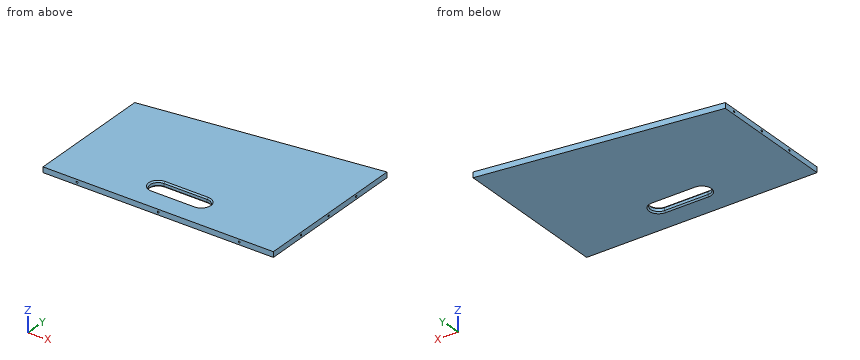
```python
from build123d import *

# Parameters (mm, degrees)
BOSS_EXTRUDE1_DEPTH       = 10
CUT_EXTRUDE1_DEPTH        = 516.437678095
CHAMFER1_SIZE             = 2.5
M4X0_7_TAPPED_HOLE1_D     = 3.3
M4X0_7_TAPPED_HOLE1_DEPTH = 12
M4X0_7_TAPPED_HOLE1_TIP   = 0.991420021
M4X0_7_TAPPED_HOLE2_D     = 3.3
M4X0_7_TAPPED_HOLE2_DEPTH = 12
M4X0_7_TAPPED_HOLE2_TIP   = 0.991420021
M4X0_7_TAPPED_HOLE3_D     = 3.3
M4X0_7_TAPPED_HOLE3_DEPTH = 12
M4X0_7_TAPPED_HOLE3_TIP   = 0.991420021


with BuildPart() as part:
    # Sketch1 → Boss-Extrude1 (new body)
    with BuildSketch(Plane.XY):
        Polygon((0, 234), (0, 290), (-426, 234), (-426, 0), (0, 0), align=None)
    extrude(amount=BOSS_EXTRUDE1_DEPTH)

    # Sketch2 → Cut-Extrude1 (cut, through all)
    with BuildSketch(Plane(origin=(0, 0, 0), x_dir=(-1, 0, 0), z_dir=(0, 0, -1))):
        with BuildLine():
            Line((173, 70), (253, 70))
            ThreePointArc((253, 70), (268, 55), (253, 40))
            Line((253, 40), (173, 40))
            ThreePointArc((173, 40), (158, 55), (173, 70))
        make_face()
    extrude(amount=-CUT_EXTRUDE1_DEPTH, mode=Mode.SUBTRACT)

    # Chamfer1
    chamfer1_edges = [part.edges().sort_by_distance(p)[0] for p in [
        (-268, 55, 10),
        (-213, 40, 10),
        (-158, 55, 10),
        (-213, 70, 10),
        (-268, 55, 0),
        (-213, 70, 0),
        (-158, 55, 0),
        (-213, 40, 0),
    ]]
    chamfer(chamfer1_edges, length=CHAMFER1_SIZE)

    # M4x0.7 Tapped Hole1
    with Locations(Plane(origin=(0, 0, 0), x_dir=(-1, 0, 0), z_dir=(0, -1, 0))):
        with Locations((63, -5), (213, -5), (363, -5)):
            Hole(M4X0_7_TAPPED_HOLE1_D / 2, depth=M4X0_7_TAPPED_HOLE1_DEPTH)
            with Locations((0, 0, -(M4X0_7_TAPPED_HOLE1_DEPTH + M4X0_7_TAPPED_HOLE1_TIP / 2))):  # 118° drill point
                Cone(0, M4X0_7_TAPPED_HOLE1_D / 2, M4X0_7_TAPPED_HOLE1_TIP, mode=Mode.SUBTRACT)

    # M4x0.7 Tapped Hole2
    with Locations(Plane.ZY.offset(426)):
        with Locations((5, 70.5), (5, 141), (5, 211.5)):
            Hole(M4X0_7_TAPPED_HOLE2_D / 2, depth=M4X0_7_TAPPED_HOLE2_DEPTH)
            with Locations((0, 0, -(M4X0_7_TAPPED_HOLE2_DEPTH + M4X0_7_TAPPED_HOLE2_TIP / 2))):  # 118° drill point
                Cone(0, M4X0_7_TAPPED_HOLE2_D / 2, M4X0_7_TAPPED_HOLE2_TIP, mode=Mode.SUBTRACT)

    # M4x0.7 Tapped Hole3
    with Locations(Plane(origin=(0, 0, 0), x_dir=(0, 0, -1), z_dir=(1, 0, 0))):
        with Locations((-5, 70.5), (-5, 141), (-5, 211.5)):
            Hole(M4X0_7_TAPPED_HOLE3_D / 2, depth=M4X0_7_TAPPED_HOLE3_DEPTH)
            with Locations((0, 0, -(M4X0_7_TAPPED_HOLE3_DEPTH + M4X0_7_TAPPED_HOLE3_TIP / 2))):  # 118° drill point
                Cone(0, M4X0_7_TAPPED_HOLE3_D / 2, M4X0_7_TAPPED_HOLE3_TIP, mode=Mode.SUBTRACT)


solid = part.part
```
Read the model definition and answer for the solid it produces. Units are mm, in the model's axes. Round coordinates to 2 decimals unless told otherwise and drop trailing zeros. Write each loop counter-clockwise with the first axis right and the second up, starting at its lowest first coordinate (ties: lowest second). Pieces come first, ordered by that corner, then holes. Notation, with made-up numbers: (19.5, -36) - (49.5, -36) arc R9 ccw to (49.5, -26) - close; hole circle Ø5 at (37.5, 28). An arc over 180 degrees is marked (long way). Use CSV: the item, a comma, the result in double quotes.
Q1. Find section A-A, the plane x = -219.5. Write down the section's boundary in (y, z), then the cut area to 3 significant figures.
Values:
outline,"(0, 0) - (37.5, 0) - (40, 2.5) - (40, 7.5) - (37.5, 10) - (0, 10) - close; (70, 2.5) - (72.5, 0) - (261.15, 0) - (261.15, 10) - (72.5, 10) - (70, 7.5) - close"
area,"2,300 mm²"
Q2. Each of these flat-tipped pins is pushed along its axis until it touches: pin 1 Ø2 at (y, z) = (211.5, 5) entering from +X; pin 2 Ø1.5 at (x, z) = (-286, 5) entering from +Y; pin 3 Ø3 at (y, z) = (70.5, 5) entering from -X. Where does it stop, or does it pass through?
Values:
pin 1,"stops at x = -12.39"
pin 2,"stops at y = 252.5"
pin 3,"stops at x = -413.91"
Q3. Straight lines are drawn through the part: line 1 along X through (y, z) = (6, 5); line 2 along Z through (x, y) = (-418, 211); line 3 along Y through (x, z) = (-4, 5). For each, find the intervals that lie inside material, in ascending order.
Values:
line 1,"x = -426 to -364.65, -361.35 to -214.65, -211.35 to -64.65, -61.35 to 0"
line 2,"z = 0 to 3.43, 6.57 to 10"
line 3,"y = 0 to 68.85, 72.15 to 139.35, 142.65 to 209.85, 213.15 to 289.47"
Q4. Find section C-C, the plane y = 249. Write down the section's boundary in (x, z).
Values:
outline,"(-311.89, 0) - (0, 0) - (0, 10) - (-311.89, 10) - close"
Q5. Find section B-B, the plane x = -116. Write down the section's boundary in (y, z), then the cut area to 3 significant figures.
Values:
outline,"(0, 0) - (274.75, 0) - (274.75, 10) - (0, 10) - close"
area,"2,750 mm²"
